CAD build for the part. Positions are in the model's coordinates, mm. A direction names the side the tool comes from. Give positions to 0.01 mm unless a question says otherwise; leave off trailing zeros. Loops run counter-clockwise (first coordinate to the right, second up) from the corner with the lowest first, then second, coordinate; pieces in that order, holes last. Notation, with made-up numbers: (62.25, -15) - (73.25, -15) arc R14 cw to (73.25, 11) - close; hole circle Ø5 at (29.5, 25). An arc over 180 degrees is marked (long way). Return JSON: item names as keys, results as strings.
from build123d import *

# Parameters (mm, degrees)
SKETCH3_R             = 38.5
SKETCH3_R_2           = 32.5
BOSS_EXTRUDE3_DEPTH   = 160
SKETCH5_R             = 36.7411
SKETCH5_R_2           = 35.6743
SKETCH5_R_3           = 34.6075
CUT_EXTRUDE1_DEPTH    = 1.4224
SKETCH5_4_R           = 45
SKETCH5_4_R_2         = 38.5
BOSS_EXTRUDE5_DEPTH   = 5
SKETCH7_R             = 1.55
CUT_EXTRUDE2_DEPTH    = 5
CUT_EXTRUDE3_START    = -80
SKETCH9_R             = 38.5
SKETCH9_R_2           = 32.5
CUT_EXTRUDE3_DEPTH    = 80
CUT_EXTRUDE6_START    = -1.4224
SKETCH5_7_R           = 36.7411
SKETCH5_7_R_2         = 35.6743
SKETCH5_7_R_3         = 34.6075
CUT_EXTRUDE6_DEPTH    = 1.4224
SKETCH10_R            = 36.7411
SKETCH10_R_2          = 34.6075
BOSS_EXTRUDE6_DEPTH   = 160
SKETCH11_R            = 36.5633
SKETCH11_R_2          = 34.4043
CUT_EXTRUDE7_DEPTH    = 1.27
CUT_EXTRUDE8_START    = -1.27
SKETCH12_R            = 36.5633
SKETCH12_R_2          = 34.4043
CUT_EXTRUDE8_DEPTH    = 1.27
SKETCH15_R            = 45
SKETCH15_R_2          = 36.5633
BOSS_EXTRUDE7_DEPTH   = 5
BOSS_EXTRUDE8_START   = -5
SKETCH16_R            = 45
SKETCH16_R_2          = 36.5633
BOSS_EXTRUDE8_DEPTH   = 5
FILLET1_R             = 0.254
M3_TAPPED_HOLE2_D     = 2.5
M3_TAPPED_HOLE2_DEPTH = 5
M3_TAPPED_HOLE2_TIP   = 0.751075774
M3_TAPPED_HOLE3_D     = 2.5
M3_TAPPED_HOLE3_DEPTH = 5
M3_TAPPED_HOLE3_TIP   = 0.751075774


with BuildPart() as part:
    # Sketch3 → Boss-Extrude3 (new body)
    with BuildSketch(Plane(origin=(0, 0, 0), x_dir=(1, 0, 0), z_dir=(0, 1, 0))):
        with Locations(Location((0, 0, 0), (0, 0, 270))):
            Circle(SKETCH3_R)
        with Locations(Location((0, 0, 0), (0, 0, 270))):
            Circle(SKETCH3_R_2, mode=Mode.SUBTRACT)
    boss_extrude3 = extrude(amount=BOSS_EXTRUDE3_DEPTH)

    # Sketch5 → Cut-Extrude1 (cut)
    # profile 1 of 2: a face of its own
    with BuildSketch(Plane.XZ):
        with Locations(Location((0, 0, 0), (0, 0, 270))):
            Circle(SKETCH5_R)
        Circle(SKETCH5_R_2, mode=Mode.SUBTRACT)
    # profile 2 of 2: a face of its own
    with BuildSketch(Plane.XZ):
        Circle(SKETCH5_R_2)
        with Locations(Location((0, 0, 0), (0, 0, 270))):
            Circle(SKETCH5_R_3, mode=Mode.SUBTRACT)
    cut_extrude1 = extrude(amount=-CUT_EXTRUDE1_DEPTH, mode=Mode.SUBTRACT)

    # Sketch5<4> → Boss-Extrude5 (add)
    with BuildSketch(Plane.XZ):
        with Locations(Location((0, 0, 0), (0, 0, 270))):
            Circle(SKETCH5_4_R)
        with Locations(Location((0, 0, 0), (0, 0, 270))):
            Circle(SKETCH5_4_R_2, mode=Mode.SUBTRACT)
    boss_extrude5 = extrude(amount=-BOSS_EXTRUDE5_DEPTH)

    # Sketch7 → Cut-Extrude2 (cut)
    with BuildSketch(Plane(origin=(0, 5, 0), x_dir=(1, 0, 0), z_dir=(0, 1, 0))):
        with Locations(Location((0, 41.75, 0), (0, 0, 270))):
            Circle(SKETCH7_R)
        with Locations(Location((29.521708115, 29.521708115, 0), (0, 0, 270))):
            Circle(SKETCH7_R)
        with Locations(Location((41.75, 0, 0), (0, 0, 270))):
            Circle(SKETCH7_R)
        with Locations(Location((29.521708115, -29.521708115, 0), (0, 0, 270))):
            Circle(SKETCH7_R)
        with Locations(Location((0, -41.75, 0), (0, 0, 270))):
            Circle(SKETCH7_R)
        with Locations(Location((-29.521708115, -29.521708115, 0), (0, 0, 270))):
            Circle(SKETCH7_R)
        with Locations(Location((-41.75, 0, 0), (0, 0, 270))):
            Circle(SKETCH7_R)
        with Locations(Location((-29.521708115, 29.521708115, 0), (0, 0, 270))):
            Circle(SKETCH7_R)
    cut_extrude2 = extrude(amount=-CUT_EXTRUDE2_DEPTH, mode=Mode.SUBTRACT)

    # Sketch9 → Cut-Extrude3 (cut)
    with BuildSketch(Plane(origin=(0, 160, 0), x_dir=(1, 0, 0), z_dir=(0, 1, 0)).offset(CUT_EXTRUDE3_START)):
        with Locations(Location((0, 0, 0), (0, 0, 90))):
            Circle(SKETCH9_R)
        with Locations(Location((0, 0, 0), (0, 0, 270))):
            Circle(SKETCH9_R_2, mode=Mode.SUBTRACT)
    extrude(amount=CUT_EXTRUDE3_DEPTH, mode=Mode.SUBTRACT)

    # Mirror7: Boss-Extrude3, Cut-Extrude1, Boss-Extrude5, Cut-Extrude2 across plane
    add(boss_extrude3.mirror(Plane.ZX.offset(80)))
    add(cut_extrude1.mirror(Plane.ZX.offset(80)), mode=Mode.SUBTRACT)
    add(boss_extrude5.mirror(Plane.ZX.offset(80)))
    add(cut_extrude2.mirror(Plane.ZX.offset(80)), mode=Mode.SUBTRACT)

    # Sketch5<7> → Cut-Extrude6 (cut)
    # profile 1 of 2: a face of its own
    with BuildSketch(Plane.XZ.offset(CUT_EXTRUDE6_START)):
        with Locations(Location((0, 0, 0), (0, 0, 270))):
            Circle(SKETCH5_7_R)
        Circle(SKETCH5_7_R_2, mode=Mode.SUBTRACT)
    # profile 2 of 2: a face of its own
    with BuildSketch(Plane.XZ.offset(CUT_EXTRUDE6_START)):
        Circle(SKETCH5_7_R_2)
        with Locations(Location((0, 0, 0), (0, 0, 270))):
            Circle(SKETCH5_7_R_3, mode=Mode.SUBTRACT)
    extrude(amount=CUT_EXTRUDE6_DEPTH, mode=Mode.SUBTRACT)

    # Sketch10 → Boss-Extrude6 (add)
    with BuildSketch(Plane(origin=(0, 160, 0), x_dir=(1, 0, 0), z_dir=(0, 1, 0))):
        Circle(SKETCH10_R)
        Circle(SKETCH10_R_2, mode=Mode.SUBTRACT)
    extrude(amount=-BOSS_EXTRUDE6_DEPTH)

    # Sketch11 → Cut-Extrude7 (cut)
    with BuildSketch(Plane(origin=(0, 160, 0), x_dir=(1, 0, 0), z_dir=(0, 1, 0))):
        with Locations(Location((0, 0, 0), (0, 0, 270))):
            Circle(SKETCH11_R)
        with Locations(Location((0, 0, 0), (0, 0, 270))):
            Circle(SKETCH11_R_2, mode=Mode.SUBTRACT)
    extrude(amount=-CUT_EXTRUDE7_DEPTH, mode=Mode.SUBTRACT)

    # Sketch12 → Cut-Extrude8 (cut)
    with BuildSketch(Plane.XZ.offset(CUT_EXTRUDE8_START)):
        with Locations(Location((0, 0, 0), (0, 0, 90))):
            Circle(SKETCH12_R)
        with Locations(Location((0, 0, 0), (0, 0, 90))):
            Circle(SKETCH12_R_2, mode=Mode.SUBTRACT)
    extrude(amount=CUT_EXTRUDE8_DEPTH, mode=Mode.SUBTRACT)

    # Sketch15 → Boss-Extrude7 (add)
    with BuildSketch(Plane(origin=(0, 160, 0), x_dir=(1, 0, 0), z_dir=(0, 1, 0))):
        with Locations(Location((0, 0, 0), (0, 0, 90))):
            Circle(SKETCH15_R)
        with Locations(Location((0, 0, 0), (0, 0, 270))):
            Circle(SKETCH15_R_2, mode=Mode.SUBTRACT)
    extrude(amount=-BOSS_EXTRUDE7_DEPTH)

    # Sketch16 → Boss-Extrude8 (add)
    with BuildSketch(Plane.XZ.offset(BOSS_EXTRUDE8_START)):
        with Locations(Location((0, 0, 0), (0, 0, 270))):
            Circle(SKETCH16_R)
        with Locations(Location((0, 0, 0), (0, 0, 90))):
            Circle(SKETCH16_R_2, mode=Mode.SUBTRACT)
    extrude(amount=BOSS_EXTRUDE8_DEPTH)

    # Fillet1
    fillet1_edges = [part.edges().sort_by_distance(p)[0] for p in [
        (0, 160, -36.5633),
        (0, 160, -34.4043),
        (0, 0, -36.5633),
        (0, 0, -34.4043),
    ]]
    fillet(fillet1_edges, radius=FILLET1_R)

    # M3 Tapped Hole2
    with Locations(Plane.XZ):
        with Locations((41, 0), (28.991378029, -28.991378029), (0, -41), (-28.991378029, -28.991378029), (-41, 0), (-28.991378029, 28.991378029), (0, 41), (28.991378029, 28.991378029), (0, 0)):
            Hole(M3_TAPPED_HOLE2_D / 2, depth=M3_TAPPED_HOLE2_DEPTH)
            with Locations((0, 0, -(M3_TAPPED_HOLE2_DEPTH + M3_TAPPED_HOLE2_TIP / 2))):  # 118° drill point
                Cone(0, M3_TAPPED_HOLE2_D / 2, M3_TAPPED_HOLE2_TIP, mode=Mode.SUBTRACT)

    # M3 Tapped Hole3
    with Locations(Plane(origin=(0, 160, 0), x_dir=(1, 0, 0), z_dir=(0, 1, 0))):
        with Locations((41, 0), (28.991378029, -28.991378029), (0, -41), (-28.991378029, -28.991378029), (-41, 0), (-28.991378029, 28.991378029), (0, 41), (28.991378029, 28.991378029), (0, 0)):
            Hole(M3_TAPPED_HOLE3_D / 2, depth=M3_TAPPED_HOLE3_DEPTH)
            with Locations((0, 0, -(M3_TAPPED_HOLE3_DEPTH + M3_TAPPED_HOLE3_TIP / 2))):  # 118° drill point
                Cone(0, M3_TAPPED_HOLE3_D / 2, M3_TAPPED_HOLE3_TIP, mode=Mode.SUBTRACT)


solid = part.part
1. Which spindle directions (+Z, -Z, +X, -X, +Y, -Y) get a long thin tool onto all of the face, cutting with end or side? Do faces 1 (the face through (10.334, 159.245, 32.816)), 2 (the face through (-36.252, 0.769, -4.76)), 3 (the face through (-13.1, 5, -36.5)). Say none if no direction does.
Values follow:
{"face 1": "+Y", "face 2": "-Y", "face 3": "none"}
2. Pull direction Y, two halves, no side cores. Call faces 4 (the face through (-37.584, 81.05, -8.346)), 5 (the face through (30.2, 160, 12.5)), 6 (the face through (-17.235, 157.535, -41.569)): +Y half, -Y half, draft (parallel to the pull), parting line (faces both ways), or undercut.
Values follow:
{"face 4": "undercut", "face 5": "+Y half", "face 6": "draft"}
3. Drop flat-ended pins along their axis: P1, Ø2, axis at x = 36, y = 32, coming from the -Z side; P2, Ø12, axis at y = 121.5, z = -15.5, coming from the -X side; P3, Ø5, axis at y = 135.5, z = 19.5, coming from the +X side. Give the stop position or say it passes through.
Values follow:
{"P1": "stops at z = -16.04", "P2": "stops at x = -37.31", "P3": "stops at x = 34.54"}
4. Cut at A-A, the plane y = 119.5. Write the cut outline in (x, z).
Values follow:
{"outline": "circle Ø77 at (0, 0); hole circle Ø65 at (0, 0)"}
5. Drill centre lines: probe 1 along Z at (x, y) = (-1.5, 102); probe 2 along X at (y, z) = (46.5, 0); probe 3 along Z at (x, y) = (-12, 85). Where is each one in solid material? Low to high.
Values follow:
{"probe 1": "z = -38.47 to -32.47, 32.47 to 38.47", "probe 2": "x = -38.5 to -32.5, 32.5 to 38.5", "probe 3": "z = -36.58 to -30.2, 30.2 to 36.58"}
